Autodesk Inventor part; units mm, degrees
ref_plane "YZ Plane" through (0, 0, 0) normal (1, 0, 0) x (0, 1, 0)
ref_plane "XZ Plane" through (0, 0, 0) normal (0, 1, 0) x (-1, 0, 0)
ref_plane "XY Plane" through (0, 0, 0) normal (0, 0, 1) x (1, 0, 0)
sketch "Sketch1" plane through (0, 0, 0) normal (0, 1, 0) x (-1, 0, 0)
  line L0 (0, 0) -> (41.148, 0)
  line L1 (41.148, 0) -> (41.148, -20.32)
  line L2 (41.148, -20.32) -> (0, -20.32)
  line L3 (0, -20.32) -> (0, 0)
  circle A0 centre (45.212, -15.24) radius 2.0193
  circle A1 centre (-4.064, -15.24) radius 2.0193
  circle A2 centre (45.212, -5.08) radius 2.0193
  circle A3 centre (-4.064, -5.08) radius 2.0193
  line L4 (41.148, -9.652) -> (49.276, -9.652)
  line L5 (41.148, -10.668) -> (49.276, -10.668)
  line L6 (-8.128, -9.652) -> (0, -9.652)
  line L7 (-8.128, -10.668) -> (0, -10.668)
  line L8 (-8.128, 3.81) -> (49.276, 3.81)
  line L9 (49.276, 3.81) -> (49.276, -24.13)
  line L10 (49.276, -24.13) -> (-8.128, -24.13)
  line L11 (-8.128, -24.13) -> (-8.128, 3.81)
  line L12 (-6.155, -5.4575) -> (-6.0508, -5.4409)
  line L13 (-6.155, -5.4575) -> (-6.0508, -5.4409)
  line L14 (20.574, -20.32) -> (20.574, 0)
  line L15 (-38.8148, -33.5345) -> (54.3929, -33.5345)
  line L16 (-38.8148, 13.2145) -> (52.2934, 13.2145)
  circle A4 centre (10.668, -10.16) radius 6.604
  point P0 (20.574, -10.16)
  dimension "d0" = 41.148
  dimension "d1" = 20.32
  dimension "d4" = 4.0386
  dimension "d5" = 4.0386
  dimension "d18" = 4.064
  dimension "d19" = 4.064
  dimension "d52" = 8.128
  dimension "d53" = 8.128
  dimension "d54" = 3.81
  dimension "d55" = 3.81
  dimension "d59" = 9.906
  dimension "d60" = 13.208
extrude "Extrusion10" add sketch "Sketch1" along normal blind 11.811
extrude "Extrusion11" cut sketch "Sketch1" along normal blind 10.16 contours L0 L14 L2 L3 | L0 L1 L2 L14
extrude "Extrusion12" cut sketch "Sketch1" along normal blind 2.032 contours L3 L7 L11 L6 | L4 L9 L5 L1
properties part number "Servo Mount"
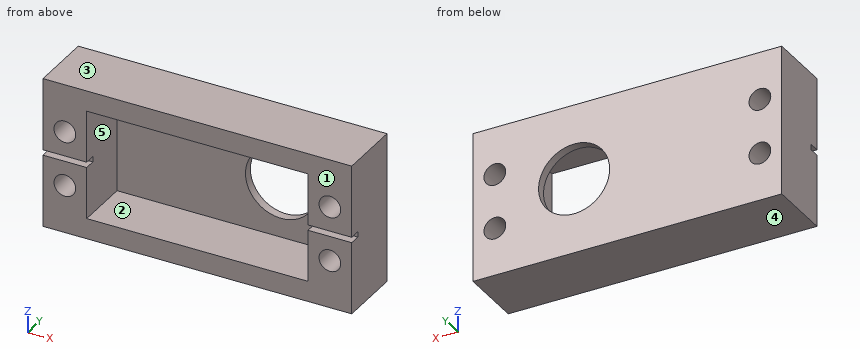
CAD build for the part. Positions are in the model's coordinates, mm. Face numbers are marked on the shaded views. A direction names the side the tool comes from. Coordinates: 2 decimals unless noted, no trailing zeros. Order: outer loops, then holes, each group sorted by start corner. A loop starts at its lowest first (then second) coordinate and runs counter-clockwise, first axis right, second up.
(1) Mould opens along Z. For the marked faces 1, 2 and 3 say: released by +Z, released by -Z, zero draft, split by the parting line, or undercut.
Solution:
face 1: zero draft
face 2: undercut
face 3: released by +Z
(2) Saw through at D-D, the plane z = -8.5. Write the cut outline in (x, y).
Solution:
outline: (-49.28, 0) - (-41.15, 0) - (-41.15, 10.16) - (-17.06, 10.16) - (-17.06, 11.81) - (-49.28, 11.81) - close; (-4.28, 10.16) - (0, 10.16) - (0, 0) - (8.13, 0) - (8.13, 11.81) - (-4.28, 11.81) - close
(3) Saw through at C-C, the plane x = 3. Write the cut outline in (y, z), and give its area (3 significant figures).
Solution:
outline: (0, -24.13) - (11.81, -24.13) - (11.81, -16.96) - (0, -16.96) - close; (0, -13.52) - (11.81, -13.52) - (11.81, -6.8) - (0, -6.8) - (0, -9.65) - (2.03, -9.65) - (2.03, -10.67) - (0, -10.67) - close; (0, -3.36) - (11.81, -3.36) - (11.81, 3.81) - (0, 3.81) - close
area: 247 mm2
(4) Drill centre lines: L1, parallel to Z at x = -2.5, y = 6; L2, parallel to X at y = 9, z = -17.75; L3, parallel to Z at x = -47, y = 1.75. Where is each one in solid material? Low to high.
Solution:
L1: z = -24.13 to -20.32, 0 to 3.81
L2: x = -49.28 to -41.15, 0 to 8.13
L3: z = -24.13 to -16.18, -14.3 to -10.67, -9.65 to -6.02, -4.14 to 3.81
(5) Saw through at A-A, the plane y = 3.25. Write the cut outline in (x, z), and give its area (4 significant figures).
Solution:
outline: (-49.28, -24.13) - (8.13, -24.13) - (8.13, 3.81) - (-49.28, 3.81) - close; hole circle Ø4.04 at (-45.21, -15.24); hole circle Ø4.04 at (-45.21, -5.08); hole (-41.15, -20.32) - (0, -20.32) - (0, 0) - (-41.15, 0) - close; hole circle Ø4.04 at (4.06, -15.24); hole circle Ø4.04 at (4.06, -5.08)
area: 716.5 mm2
(6) Pin check, flat tip, straight feed: pin 1 Ø1.5 at (x, z) = (-12.5, -18) entering from -Y. Stop position of the tip, or through.
Solution:
pin 1: stops at y = 10.16
(7) Saw through at B-B, the plane z = -15.24. Write the cut outline in (x, y), and give its area (3 significant figures).
Solution:
outline: (-49.28, 0) - (-47.23, 0) - (-47.23, 11.81) - (-49.28, 11.81) - close; (-43.19, 0) - (-41.15, 0) - (-41.15, 10.16) - (-14.89, 10.16) - (-14.89, 11.81) - (-43.19, 11.81) - close; (-6.45, 10.16) - (0, 10.16) - (0, 0) - (2.04, 0) - (2.04, 11.81) - (-6.45, 11.81) - close; (6.08, 0) - (8.13, 0) - (8.13, 11.81) - (6.08, 11.81) - close
area: 151 mm2
(8) Which spindle directions (+Z, -Z, +X, -X, +Y, -Y) get a long thin tool onto all of the face, cutting with end or side? Do the marked faces 4 and 5. Say none if no direction does.
Solution:
face 4: -Z, +X, -X, +Y, -Y
face 5: -Y
